Geometry check sheet. Reference: the model listing, model coordinates, mm. A direction names the side the tool comes from. Give positions to 0.01 mm unless a question says otherwise; leave off trailing zeros. Loops run counter-clockwise (first coordinate to the right, second up) from the corner with the lowest first, then second, coordinate; pieces in that order, holes last. Notation, with made-up numbers: (-14, -1.75) -> (34, -1.75) arc R16 ccw to (34, 18.25) -> close; hole circle Ø5 at (88.5, 89). An arc over 180 degrees is marked (long way). One line per item, written item: value. Start each with the question number.
(1) Tool access check on faces 4 (the face through (-4.575, -3.021, 13.655)), 5 (the face through (-39, -7.509, 12)), 6 (the face through (-21, -10, -14)). Record the directions out of +Z, -Z, +X, -X, +Y, -Y that give a thin tool (end or side, any length) a straight path to the whole face; none if there is none.
(2) Sectioned sample at C-C, the plane y = 0.5. Record the cut outline in (x, z), then the cut area to 3 significant figures.
(3) Sectioned sample at A-A, the plane z = -13.5. Record the cut outline in (x, y), then the cut area to 3 significant figures.
(4) Draft check along Z on faces 1 (the face through (-40.111, -3.8, 13.3)), 2 (the face through (-21, -10, -16)), 3 (the face through (-37.19, -4.06, -14.99)). Enter one of: pulls with the +Z half, pulls with the -Z half, needs draft (parallel to the pull), parting line crosses it, or undercut.
(5) Gauge pin test, flat end, axial feed: pin 1 Ø3.5 at (x, y) = (-4.38, -15.49) entering from -Z. Record the tip position at first contact, or that the pin passes through.
(6) Sectioned sample at B-B, the plane x = -4.38. State how many separate pieces and enclosed holes the cut face has, then the cut area to 3 significant figures.
(7) Scan lines: line 1 along Y through (x, z) = (-38.62, -14.85); line 2 along Y through (x, z) = (-3, -12); line 3 along Z through (x, y) = (-13, -6). Record each from-to range of solid material in increasing order. Write a range as from..to.
(8) Sectioned sample at D-D, the plane x = -19.5. Record the cut outline in (y, z), then the cut area to 3 significant figures.
from build123d import *

# Parameters (mm, degrees)
SKETCH19_W          = 30
SKETCH19_H          = 28
SKETCH19_W_2        = 25
SKETCH19_H_2        = 22
BOSS_EXTRUDE1_DEPTH = 43
SKETCH30_R          = 1.5
CUT_EXTRUDE2_DEPTH  = 31
CUT_EXTRUDE4_DEPTH  = 2.3


with BuildPart() as part:
    # Sketch19 → Boss-Extrude1 (new body)
    with BuildSketch(Plane(origin=(0, 0, 0), x_dir=(0, 0, -1), z_dir=(1, 0, 0))):
        with Locations((1, -10)):
            Rectangle(SKETCH19_W, SKETCH19_H)
        with Locations((1.5, -10)):
            Rectangle(SKETCH19_W_2, SKETCH19_H_2, mode=Mode.SUBTRACT)
    extrude(amount=-BOSS_EXTRUDE1_DEPTH)

    # Sketch30 → Cut-Extrude2 (cut, through all)
    with BuildSketch(Plane.XY.offset(14)):
        with Locations((-38.62, -4.508713144)):
            Circle(SKETCH30_R)
        with Locations((-4.38, -4.508713144)):
            Circle(SKETCH30_R)
        with Locations((-4.38, -15.491286856)):
            Circle(SKETCH30_R)
        with Locations((-38.62, -15.491286856)):
            Circle(SKETCH30_R)
    extrude(amount=-CUT_EXTRUDE2_DEPTH, mode=Mode.SUBTRACT)

    # Sketch31 → Cut-Extrude4 (cut)
    with BuildSketch(Plane(origin=(0, 0, 11), x_dir=(-1, 0, 0), z_dir=(0, 0, -1))):
        Polygon((42.084101615, -4.508713144), (40.352050808, -1.508713144), (36.887949192, -1.508713144), (35.155898385, -4.508713144), (36.887949192, -7.508713144), (40.352050808, -7.508713144), align=None)
        Polygon((7.844101615, -4.508713144), (6.112050808, -1.508713144), (2.647949192, -1.508713144), (0.915898385, -4.508713144), (2.647949192, -7.508713144), (6.112050808, -7.508713144), align=None)
        Polygon((7.844101615, -15.491286856), (6.112050808, -12.491286856), (2.647949192, -12.491286856), (0.915898385, -15.491286856), (2.647949192, -18.491286856), (6.112050808, -18.491286856), align=None)
        Polygon((42.084101615, -15.491286856), (40.352050808, -12.491286856), (36.887949192, -12.491286856), (35.155898385, -15.491286856), (36.887949192, -18.491286856), (40.352050808, -18.491286856), align=None)
    extrude(amount=-CUT_EXTRUDE4_DEPTH, mode=Mode.SUBTRACT)


solid = part.part
Calculated:
1. face 4: +Z, -Z
1. face 5: none
1. face 6: +X, -X
2. outline: (-43, -16) -> (0, -16) -> (0, -14) -> (-43, -14) -> close; (-43, 11) -> (0, 11) -> (0, 14) -> (-43, 14) -> close
2. area: 215 mm2
3. outline: (-43, -24) -> (0, -24) -> (0, -21) -> (-43, -21) -> close; (-43, 1) -> (0, 1) -> (0, 4) -> (-43, 4) -> close
3. area: 258 mm2
4. face 1: undercut
4. face 2: pulls with the -Z half
4. face 3: needs draft
5. pin 1: stops at z = -16
6. separate pieces: 4
6. enclosed holes: 0
6. area: 246 mm2
7. line 1: y = -24..-16.99, -13.99..-6.01, -3.01..4
7. line 2: y = -24..-21, 1..4
7. line 3: z = -16..-14, 11..14
8. outline: (-24, -16) -> (4, -16) -> (4, 14) -> (-24, 14) -> close; hole (-21, -14) -> (1, -14) -> (1, 11) -> (-21, 11) -> close
8. area: 290 mm2
